from build123d import *

# Parameters (mm, degrees)
SKETCH1_W           = 50
SKETCH1_H           = 26
SKETCH1_R           = 1.55
BOSS_EXTRUDE1_DEPTH = 3
SKETCH2_W           = 29
SKETCH2_H           = 26
SKETCH2_R           = 1.55
BOSS_EXTRUDE2_DEPTH = 3
BOSS_EXTRUDE3_START = -47
SKETCH2_2_W         = 29
SKETCH2_2_H         = 26
SKETCH2_2_R         = 1.55
BOSS_EXTRUDE3_DEPTH = 3
BOSS_EXTRUDE4_DEPTH = 3
BOSS_EXTRUDE5_START = -26
BOSS_EXTRUDE5_DEPTH = 3


with BuildPart() as part:
    # Sketch1 → Boss-Extrude1 (new body)
    with BuildSketch(Plane.XY):
        Rectangle(SKETCH1_W, SKETCH1_H)
        with Locations((-7, 0)):
            Circle(SKETCH1_R, mode=Mode.SUBTRACT)
        with Locations((0, 7)):
            Circle(SKETCH1_R, mode=Mode.SUBTRACT)
        with Locations((7, 0)):
            Circle(SKETCH1_R, mode=Mode.SUBTRACT)
        with Locations((0, -7)):
            Circle(SKETCH1_R, mode=Mode.SUBTRACT)
    extrude(amount=BOSS_EXTRUDE1_DEPTH)

    # Sketch2 → Boss-Extrude2 (add)
    with BuildSketch(Plane.ZY.offset(25)):
        with Locations((-11.5, 0)):
            Rectangle(SKETCH2_W, SKETCH2_H)
        with Locations((-4.5, 0)):
            Circle(SKETCH2_R, mode=Mode.SUBTRACT)
        with Locations((-13, -8.5)):
            Circle(SKETCH2_R, mode=Mode.SUBTRACT)
        with Locations((-21.5, 0)):
            Circle(SKETCH2_R, mode=Mode.SUBTRACT)
        with Locations((-13, 8.5)):
            Circle(SKETCH2_R, mode=Mode.SUBTRACT)
    extrude(amount=-BOSS_EXTRUDE2_DEPTH)

    # Sketch2<2> → Boss-Extrude3 (add)
    with BuildSketch(Plane.ZY.offset(25).offset(BOSS_EXTRUDE3_START)):
        with Locations((-11.5, 0)):
            Rectangle(SKETCH2_2_W, SKETCH2_2_H)
        with Locations((-4.5, 0)):
            Circle(SKETCH2_2_R, mode=Mode.SUBTRACT)
        with Locations((-13, -8.5)):
            Circle(SKETCH2_2_R, mode=Mode.SUBTRACT)
        with Locations((-21.5, 0)):
            Circle(SKETCH2_2_R, mode=Mode.SUBTRACT)
        with Locations((-13, 8.5)):
            Circle(SKETCH2_2_R, mode=Mode.SUBTRACT)
    extrude(amount=-BOSS_EXTRUDE3_DEPTH)

    # Sketch3 → Boss-Extrude4 (add)
    with BuildSketch(Plane(origin=(0, 13, 0), x_dir=(1, 0, 0), z_dir=(0, 1, 0))):
        Polygon((-25, -3), (-25, 11.5), (-13.5, 0), (13.5, 0), (25, 11.5), (25, -3), align=None)
    extrude(amount=BOSS_EXTRUDE4_DEPTH)

    # Sketch3<3> → Boss-Extrude5 (add)
    with BuildSketch(Plane(origin=(0, 13, 0), x_dir=(1, 0, 0), z_dir=(0, 1, 0)).offset(BOSS_EXTRUDE5_START)):
        Polygon((-25, -3), (-25, 11.5), (-13.5, 0), (13.5, 0), (25, 11.5), (25, -3), align=None)
    extrude(amount=-BOSS_EXTRUDE5_DEPTH)


solid = part.part
Source: CAD feature listing. Evaluate the final solid. Frame: model axes, mm. A direction names the side the tool comes from. Give positions to 0.01 mm unless a question says otherwise; leave off trailing zeros. Loops run counter-clockwise (first coordinate to the right, second up) from the corner with the lowest first, then second, coordinate; pieces in that order, holes last. Notation, with made-up numbers: (46, 43.25) -> (51, 43.25) arc R21 cw to (51, 77.25) -> close; hole circle Ø7 at (37, 64.25). An arc over 180 degrees is marked (long way). Use a Markdown table: item, result. Add a question column.
1) Section query D-D, the plane z = -21.5. Return the cut outline in (x, y), then the cut area to 3 significant figures.
2) Pull-direction query (Z, two-part tool) for faces 1 (the face through (-19.3, -14.5, -5.8)), 2 (the face through (-0.336, -8.513, 1.479)), 3 (the face through (-23.521, -0.594, -20.068)), 4 (the face through (-23.52, 0.07, -6.05)); classes: +Z half, -Z half, draft (parallel to the pull), parting line (faces both ways), or undercut.
3) Section query A-A, the plane z = -13. Return the cut outline in (x, y).
4) Reachability of faces 5 (the face through (-23.52, 7.56, -14.23)), 6 (the face through (-22, 0, -13)) from +Z, -Z, +X, -X, +Y, -Y: full face, straight path, thin tool, end or side. Return the list, or none.
5) Section query C-C, the plane y = 0. Count the separate pieces of the cut face and the enclosed holes in it, then the cut area to 3 significant figures.
6) First-contact query: pin 1 (4 mm diameter, centred on x = 19.5, z = -6.5, fed in from +Y); pin 2 (2.5 mm diameter, centred on x = 23.5, z = -15.5, fed in from -Y); pin 3 (12 mm diameter, centred on x = -10.5, y = -6.5, fed in from -Z); pin 4 (0.9 mm diameter, centred on x = -23, z = -17.5, fed in from +Y). Flat tips, straight axial feed; report the tip coordinate or a pass-through.
7) Section query B-B, the plane x = 7. Return the cut outline in (y, z), then the cut area to 3 significant figures.
8) Line query: line 1 along Y through (x, z) = (23.4, -13); line 2 along Y through (x, z) = (0, 2.4); line 3 along X through (y, z) = (2, -20). Output: solid intervals per line, ascending. Write a range as [from, to].
Numbers:
| question | item | result |
|---|---|---|
| 1 | outline | (-25, -13) -> (-22, -13) -> (-22, -1.55) -> (-25, -1.55) -> close; (-25, 1.55) -> (-22, 1.55) -> (-22, 13) -> (-25, 13) -> close; (22, -13) -> (25, -13) -> (25, -1.55) -> (22, -1.55) -> close; (22, 1.55) -> (25, 1.55) -> (25, 13) -> (22, 13) -> close |
| 1 | area | 137 mm2 |
| 2 | face 1 | -Z half |
| 2 | face 2 | draft |
| 2 | face 3 | undercut |
| 2 | face 4 | undercut |
| 3 | outline | (-25, -13) -> (-22, -13) -> (-22, -10.05) -> (-25, -10.05) -> close; (-25, -6.95) -> (-22, -6.95) -> (-22, 6.95) -> (-25, 6.95) -> close; (-25, 10.05) -> (-22, 10.05) -> (-22, 13) -> (-25, 13) -> close; (22, -13) -> (25, -13) -> (25, -10.05) -> (22, -10.05) -> close; (22, -6.95) -> (25, -6.95) -> (25, 6.95) -> (22, 6.95) -> close; (22, 10.05) -> (25, 10.05) -> (25, 13) -> (22, 13) -> close |
| 4 | face 5 | +X, -X |
| 4 | face 6 | -Z |
| 5 | separate pieces | 7 |
| 5 | enclosed holes | 0 |
| 5 | area | 250 mm2 |
| 6 | pin 1 | stops at y = 16 |
| 6 | pin 2 | stops at y = -13 |
| 6 | pin 3 | stops at z = 0 |
| 6 | pin 4 | stops at y = 13 |
| 7 | outline | (-16, 0) -> (-1.55, 0) -> (-1.55, 3) -> (-16, 3) -> close; (1.55, 0) -> (16, 0) -> (16, 3) -> (1.55, 3) -> close |
| 7 | area | 86.7 mm2 |
| 8 | line 1 | y = [-13, -10.05], [-6.95, 6.95], [10.05, 13] |
| 8 | line 2 | y = [-16, -8.55], [-5.45, 5.45], [8.55, 16] |
| 8 | line 3 | x = [-25, -22], [22, 25] |
